Input: part model. Units: mm. Frame: model coordinates. Give positions to 0.01 mm unless a question says otherwise; leave off trailing zeros. Loops run counter-clockwise (first coordinate to the right, second up) from the corner with the lowest first, then second, coordinate; pieces in that order, holes last. Notation, with made-up numbers: (88.25, 68) -> (102.25, 68) arc R8 cw to (102.25, 74) -> close; hole circle Ø5 at (73, 26.5). An arc over 180 degrees is marked (long way). One line per question, with ' | ' between items.
from build123d import *

# Parameters (mm, degrees)
SKETCH_1_W             = 61
SKETCH_1_H             = 91
EXTRUDE_1_DEPTH        = 35
HOLE_WIZARD_M3_1_D     = 2.5
HOLE_WIZARD_M3_1_DEPTH = 10
HOLE_WIZARD_M3_1_TIP   = 0.751075774
M3X0_5_1_D             = 2.5
M3X0_5_1_DEPTH         = 10
M3X0_5_1_TIP           = 0.751075774
HOLE_WIZARD_M3_2_D     = 2.5
HOLE_WIZARD_M3_2_DEPTH = 10
HOLE_WIZARD_M3_2_TIP   = 0.751075774
FILLET_1_R             = 1
SKETCH_9_W             = 7.285769401
SKETCH_9_H             = 3.095672023
CUT_EXTRUDE_1_DEPTH    = 10
SKETCH_10_W            = 75.598284418
SKETCH_10_H            = 3.429789841
CUT_EXTRUDE_2_DEPTH    = 10


with BuildPart() as part:
    # 草图1 → 凸台-拉伸1 (new body)
    with BuildSketch(Plane(origin=(0, 0, 0), x_dir=(1, 0, 0), z_dir=(0, 1, 0))):
        Rectangle(SKETCH_1_W, SKETCH_1_H)
    extrude(amount=EXTRUDE_1_DEPTH)

    # M3 螺纹孔1
    with Locations(Plane(origin=(-22.5, 3, 45.5), x_dir=(1, 0, 0), z_dir=(0, 0, 1))):
        with Locations((0, 0), (45, 0)):
            Hole(HOLE_WIZARD_M3_1_D / 2, depth=HOLE_WIZARD_M3_1_DEPTH)
            with Locations((0, 0, -(HOLE_WIZARD_M3_1_DEPTH + HOLE_WIZARD_M3_1_TIP / 2))):  # 118° drill point
                Cone(0, HOLE_WIZARD_M3_1_D / 2, HOLE_WIZARD_M3_1_TIP, mode=Mode.SUBTRACT)

    # M3x0.5 螺纹孔1
    with Locations(Plane(origin=(0, 0, -45.5), x_dir=(-1, 0, 0), z_dir=(0, 0, -1))):
        with Locations((-22.5, 3), (22.5, 3)):
            Hole(M3X0_5_1_D / 2, depth=M3X0_5_1_DEPTH)
            with Locations((0, 0, -(M3X0_5_1_DEPTH + M3X0_5_1_TIP / 2))):  # 118° drill point
                Cone(0, M3X0_5_1_D / 2, M3X0_5_1_TIP, mode=Mode.SUBTRACT)

    # M3 螺纹孔2
    with Locations(Plane(origin=(0, 0, 0), x_dir=(-1, 0, 0), z_dir=(0, -1, 0))):
        with Locations((14, 0), (-14, 0)):
            Hole(HOLE_WIZARD_M3_2_D / 2, depth=HOLE_WIZARD_M3_2_DEPTH)
            with Locations((0, 0, -(HOLE_WIZARD_M3_2_DEPTH + HOLE_WIZARD_M3_2_TIP / 2))):  # 118° drill point
                Cone(0, HOLE_WIZARD_M3_2_D / 2, HOLE_WIZARD_M3_2_TIP, mode=Mode.SUBTRACT)

    # 圆角1
    fillet_1_edges = [part.edges().sort_by_distance(p)[0] for p in [
        (-30.5, 35, 0),
        (0, 35, 45.5),
        (30.5, 35, 0),
        (0, 0, 45.5),
        (-30.5, 0, 0),
        (0, 0, -45.5),
        (30.5, 0, 0),
        (30.5, 17.5, 45.5),
        (-30.5, 17.5, 45.5),
        (-30.5, 17.5, -45.5),
        (30.5, 17.5, -45.5),
        (0, 35, -45.5),
    ]]
    fillet(fillet_1_edges, radius=FILLET_1_R)

    # 草图9 → 切除-拉伸1 (cut)
    with BuildSketch(Plane.XY.offset(45.5)):
        with Locations((14.053983322, 6.612378958)):
            Rectangle(SKETCH_9_W, SKETCH_9_H)
        with Locations((-14.053983322, 6.612378958)):
            Rectangle(SKETCH_9_W, SKETCH_9_H)
    extrude(amount=-CUT_EXTRUDE_1_DEPTH, mode=Mode.SUBTRACT)

    # 草图10 → 切除-拉伸2 (cut)
    with BuildSketch(Plane.ZY.offset(30.5)):
        with Locations((0, 4.995557871)):
            Rectangle(SKETCH_10_W, SKETCH_10_H)
    extrude(amount=-CUT_EXTRUDE_2_DEPTH, mode=Mode.SUBTRACT)


solid = part.part
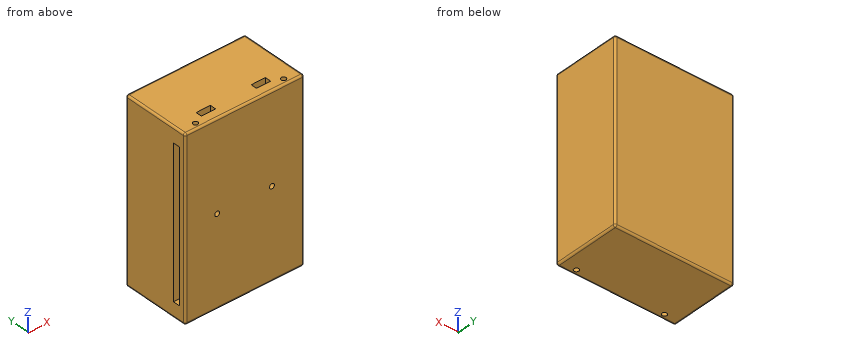
1. Ray query, line 1 along X through (y, z) = (3, 43); line 2 along Y through (x, z) = (-22.5, 30.5); line 3 along Y through (x, z) = (-22.5, -40.5). Return the intervals inside material, ascending. Write a range as from..to.
Determined:
line 1: x = -30.5..-23.75, -21.25..21.25, 23.75..30.5 | line 2: y = 0..3.28, 6.71..35 | line 3: y = 0..1.75, 4.25..35
2. Section query A-A (z = -22.5). Output: boundary loops of the cut face in (x, y).
Determined:
outline: (-30.5, 1) arc R1 ccw to (-29.5, 0) -> (29.5, 0) arc R1 ccw to (30.5, 1) -> (30.5, 34) arc R1 ccw to (29.5, 35) -> (-29.5, 35) arc R1 ccw to (-30.5, 34) -> (-30.5, 6.71) -> (-20.5, 6.71) -> (-20.5, 3.28) -> (-30.5, 3.28) -> close
3. Pin query (flat end, axial travel): P1, Ø2, axis at x = -22.5, y = 3, coming from the -Z side; P2, Ø1.5, axis at x = -15.5, y = 6.5, coming from the +Z side; P3, Ø2, axis at x = -22.5, y = 3, coming from the +Z side. Return the tip coordinate at first contact, or that it passes through.
Determined:
P1: stops at z = -35.35 | P2: stops at z = 35.5 | P3: stops at z = 35.35
